from build123d import *

# Parameters (mm, degrees)
F1_DEPTH = 25.4


# Not quite as in the source:
# - a feature names something its author has since deleted; it is built from what else it names


with BuildPart() as f1:
    # F0 (on Front) → F1 (new body)
    with BuildSketch(Plane.XZ):
        with BuildLine():
            ThreePointArc((-38.9001, 29.1195621888), (-31.75, 36.2696621888), (-24.5999, 29.1195621888))
            ThreePointArc((-24.5999, 29.1195621888), (-26.0973866941, 24.7409901814), (-29.9625922208, 22.1964773676))
            Line((-29.9625922208, 22.1964773676), (-28.5752082075, 16.8227863075))
            ThreePointArc((-28.5752082075, 16.8227863075), (-21.7098342702, 21.3423472555), (-19.05, 29.1195621888))
            ThreePointArc((-19.05, 29.1195621888), (-19.0991685805, 30.2360138876), (-19.2462936057, 31.3438208077))
            Line((-19.2462936057, 31.3438208077), (-19.7336528982, 33.2302071905))
            ThreePointArc((-19.7336528982, 33.2302071905), (-33.8335536719, 41.6474831694), (-44.45, 29.1195621888))
            Line((-44.45, 29.1195621888), (-38.9001, 29.1195621888))
        make_face()
        with BuildLine():
            ThreePointArc((-29.9625922208, 22.1964773676), (-36.1285720074, 23.4669488829), (-38.9001, 29.1195621888))
            Line((-38.9001, 29.1195621888), (-44.45, 29.1195621888))
            ThreePointArc((-44.45, 29.1195621888), (-44.3685455909, 27.683488663), (-44.1252272171, 26.2658363215))
            Line((-44.1252272171, 26.2658363215), (-43.9599962271, 25.6258546831))
            ThreePointArc((-43.9599962271, 25.6258546831), (-38.0573158317, 18.0965060336), (-28.5752082075, 16.8227863075))
            Line((-28.5752082075, 16.8227863075), (-29.9625922208, 22.1964773676))
        make_face()
        with BuildLine():
            Line((28.5710442304, -204.5191802253), (-28.5752082075, 16.8227863075))
            ThreePointArc((-28.5752082075, 16.8227863075), (-38.0573158317, 18.0965060336), (-43.9599962271, 25.6258546831))
            Line((-43.9599962271, 25.6258546831), (18.6335537415, -216.8148802954))
            Line((18.6335537415, -216.8148802954), (19.05, -216.8148802954))
            ThreePointArc((19.05, -216.8148802954), (21.7085175827, -209.039365466), (28.5710442304, -204.5191802253))
        make_face()
        with BuildLine():
            ThreePointArc((-19.05, 29.1195621888), (-21.7098342702, 21.3423472555), (-28.5752082075, 16.8227863075))
            Line((-28.5752082075, 16.8227863075), (28.5710442304, -204.5191802253))
            ThreePointArc((28.5710442304, -204.5191802253), (38.1974658289, -205.8732083763), (44.0462542776, -213.6380688845))
            Line((44.0462542776, -213.6380688845), (18.8073706418, -115.9477465067))
            Line((18.8073706418, -115.9477465067), (11.8328057084, -88.9518022083))
            Line((11.8328057084, -88.9518022083), (9.4897628664, -79.8827556578))
            Line((9.4897628664, -79.8827556578), (-19.2462936057, 31.3438208077))
            ThreePointArc((-19.2462936057, 31.3438208077), (-19.0991685805, 30.2360138876), (-19.05, 29.1195621888))
        make_face()
        with BuildLine():
            Line((29.958428385, -209.8928718327), (28.5710442304, -204.5191802253))
            ThreePointArc((28.5710442304, -204.5191802253), (21.7085175827, -209.039365466), (19.05, -216.8148802954))
            Line((19.05, -216.8148802954), (24.5999, -216.8148802954))
            ThreePointArc((24.5999, -216.8148802954), (26.0960701183, -212.4380084784), (29.958428385, -209.8928718327))
        make_face()
        with BuildLine():
            ThreePointArc((44.0462542776, -213.6380688845), (38.1974658289, -205.8732083763), (28.5710442304, -204.5191802253))
            Line((28.5710442304, -204.5191802253), (29.958428385, -209.8928718327))
            ThreePointArc((29.958428385, -209.8928718327), (36.126871817, -211.1609504137), (38.9001, -216.8148802954))
            ThreePointArc((38.9001, -216.8148802954), (37.4012962188, -221.1951520972), (33.5332432967, -223.7390389703))
            Line((33.5332432967, -223.7390389703), (34.9206274513, -229.1127305777))
            ThreePointArc((34.9206274513, -229.1127305777), (41.7888487545, -224.5937951095), (44.45, -216.8148802954))
            ThreePointArc((44.45, -216.8148802954), (44.3486592407, -215.2136978145), (44.0462542776, -213.6380688845))
        make_face()
        with BuildLine():
            Line((24.5999, -216.8148802954), (19.05, -216.8148802954))
            ThreePointArc((19.05, -216.8148802954), (19.1512093102, -218.4150281492), (19.4532241187, -219.9896720879))
            ThreePointArc((19.4532241187, -219.9896720879), (25.2979309254, -227.7538384111), (34.9206274513, -229.1127305777))
            Line((34.9206274513, -229.1127305777), (33.5332432967, -223.7390389703))
            ThreePointArc((33.5332432967, -223.7390389703), (27.3697281982, -222.4661765142), (24.5999, -216.8148802954))
        make_face()
        Polygon((11.8328057084, -88.9518022083), (18.8073706418, -115.9477465067), (120.7016461253, -115.9477465067), (120.7016461253, -88.9518022083), align=None)
    extrude(amount=F1_DEPTH)


solid = f1.part
Source: CAD feature listing. Evaluate the final solid. Frame: model axes, mm. A direction names the side the tool comes from. Coordinates: 2 decimals unless noted, no trailing zeros. Loops run counter-clockwise (first coordinate to the right, second up) from the corner with the lowest first, then second, coordinate; pieces in that order, holes last. Notation, with made-up numbers: (22.25, 73.5) - (42.25, 73.5) arc R15 ccw to (42.25, 102.5) - close; hole circle Ø10 at (-34.75, -30.75). An arc over 180 degrees is marked (long way). One line per question, with ' | ' between items.
1) Line query: line 1 along Z through (x, y) = (106, -6.25); line 2 along X through (y, z) = (-7, -68); line 3 along X through (y, z) = (-13, -110.5). Output: solid intervals per line, ascending.
Report:
line 1: z = -115.95 to -88.95 | line 2: x = -19.79 to 6.42 | line 3: x = -8.81 to 120.7
2) First-contact query: P1, Ø7.5, axis at x = 86.5, y = -16.5, coming from the -Z side; P2, Ø13, axis at x = 31.75, z = -216.81, coming from the -Y side; P3, Ø12.5, axis at x = 74.5, y = -9, coming from the +Z side; P4, Ø6, axis at y = -19.5, z = -66.5, coming from the -X side. Flat tips, straight axial feed; report the tip coordinate or a pass-through.
Report:
P1: stops at z = -115.95 | P2: passes through | P3: stops at z = -88.95 | P4: stops at x = -20.95
3) Set-up query: faces 4 (the face through (69, -13, -115.948)), 5 (the face through (120.702, -13, -103)). Return all of +Z, -Z, +X, -X, +Y, -Y with unobstructed straight access to the full face (end or side cutting, diameter ignored); none if empty.
Report:
face 4: +X, +Y, -Y | face 5: +Z, -Z, +X, +Y, -Y
4) Section B-B, the plane z = -197.5. Return loops of the section in (x, y).
Report:
outline: (13.65, -25.4) - (39.88, -25.4) - (39.88, 0) - (13.65, 0) - close
5) Section A-A, the plane y = -14. Return loops of the section in (x, z).
Report:
outline: (-44.13, 26.27) - (18.63, -216.81) - (19.05, -216.81) arc R12.7 ccw (long way) to (44.05, -213.64) - (18.81, -115.95) - (120.7, -115.95) - (120.7, -88.95) - (11.83, -88.95) - (-19.73, 33.23) arc R12.7 ccw to start; hole circle Ø14.3 at (-31.75, 29.12); hole circle Ø14.3 at (31.75, -216.81)
6) Pull-direction query (Z, two-part tool) for faces 1 (the face through (67, -13, -88.952)), 2 (the face through (13, 0, -93)), 3 (the face through (31.603, -12.522, -165.477)); classes: released by +Z, released by -Z, zero draft, split by the parting line, or undercut.
Report:
face 1: released by +Z | face 2: zero draft | face 3: undercut
7) Section C-C, the plane z = 12. Return loops of the section in (x, y), then the cut area to 3 significant figures.
Report:
outline: (-40.44, -25.4) - (-14.25, -25.4) - (-14.25, 0) - (-40.44, 0) - close | area: 665 mm²
